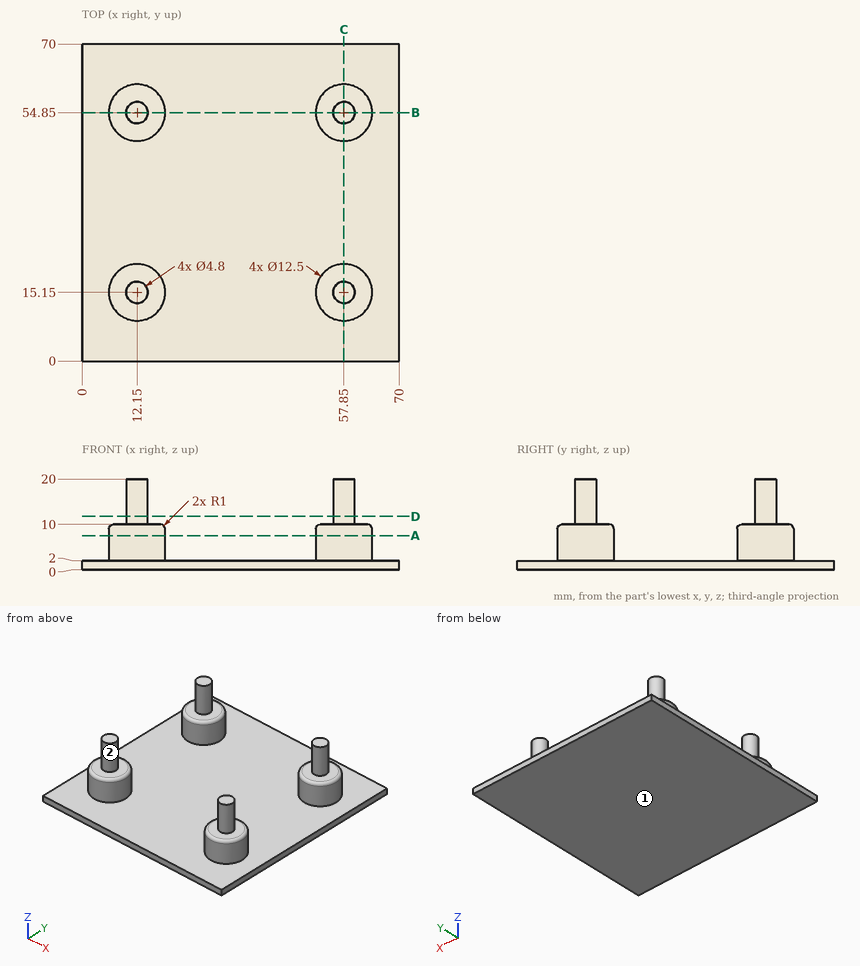
Part print with two shaded views. Sizes in mm from the minimum x, y, z corner. Give positions to 0.01 mm unless a question says otherwise; leave off trailing zeros. Order: outer loops, then holes, each group sorted by start corner. A loop starts at its lowest first (then second) coordinate and runs counter-clockwise, first axis right, second up.
(1) Saw through at B-B, the plane y = 54.85. Give the cut face in (x, z), then the cut area to 3 significant figures.
(2) Saw through at A-A, the plane z = 7.5. Give the cut face in (x, y).
(3) Flat gauge pins, fed straight in: pin 1 (2 mm diameter, centred on x = 53.5, z = 13, fed in from +Y); pin 2 (3 mm diameter, centred on y = 18.5, z = 12, fed in from +X). Where does each tip first touch, or does it go through?
(4) Saw through at D-D, the plane z = 11.75. Give the cut face in (x, y).
(5) Drill centre lines: L1, parallel to Z at x = 11.5, y = 7; L2, parallel to X at y = 10, z = 5; L3, parallel to Y at x = 10.5, z = 17.75. Where is each one in solid material? Low to high.
(6) Saw through at C-C, the plane x = 57.85. Give the cut face in (y, z), then the cut area to 3 significant figures.
(7) Mould opens along X. For the marked faces 1 and 2 say: released by +X, released by -X, zero draft, split by the parting line, or undercut.
Results found:
1. outline: (0, 0) - (70, 0) - (70, 2) - (64.1, 2) - (64.1, 9) arc R1 ccw to (63.1, 10) - (60.25, 10) - (60.25, 20) - (55.45, 20) - (55.45, 10) - (52.6, 10) arc R1 ccw to (51.6, 9) - (51.6, 2) - (18.4, 2) - (18.4, 9) arc R1 ccw to (17.4, 10) - (14.55, 10) - (14.55, 20) - (9.75, 20) - (9.75, 10) - (6.9, 10) arc R1 ccw to (5.9, 9) - (5.9, 2) - (0, 2) - close
1. area: 435 mm2
2. outline: circle Ø12.5 at (12.15, 15.15); circle Ø12.5 at (12.15, 54.85); circle Ø12.5 at (57.85, 15.15); circle Ø12.5 at (57.85, 54.85)
3. pin 1: passes through
3. pin 2: stops at x = 59.38
4. outline: circle Ø4.8 at (12.15, 15.15); circle Ø4.8 at (12.15, 54.85); circle Ø4.8 at (57.85, 15.15); circle Ø4.8 at (57.85, 54.85)
5. L1: z = 0 to 2
5. L2: x = 8.61 to 15.69, 54.31 to 61.39
5. L3: y = 13.41 to 16.89, 53.11 to 56.59
6. outline: (0, 0) - (70, 0) - (70, 2) - (61.1, 2) - (61.1, 9) arc R1 ccw to (60.1, 10) - (57.25, 10) - (57.25, 20) - (52.45, 20) - (52.45, 10) - (49.6, 10) arc R1 ccw to (48.6, 9) - (48.6, 2) - (21.4, 2) - (21.4, 9) arc R1 ccw to (20.4, 10) - (17.55, 10) - (17.55, 20) - (12.75, 20) - (12.75, 10) - (9.9, 10) arc R1 ccw to (8.9, 9) - (8.9, 2) - (0, 2) - close
6. area: 435 mm2
7. face 1: zero draft
7. face 2: undercut
